Could you check a few things on this drawing? It's one solid part, dimensions in mm from its lowest x, y, z. A direction names the side the tool comes from. Give positions to 0.01 mm unless a question says otherwise; leave off trailing zeros. Loops run counter-clockwise (first coordinate to the right, second up) from the corner with the lowest first, then second, coordinate; pieces in that order, holes last. Notation, with made-up numbers: (16, -9) - (57, -9) arc R21 cw to (57, 28) - close; hole circle Ø5 at (11.5, 28). An arc over 180 degrees is marked (long way). Use CSV: the item, a comma, the result in double quotes.
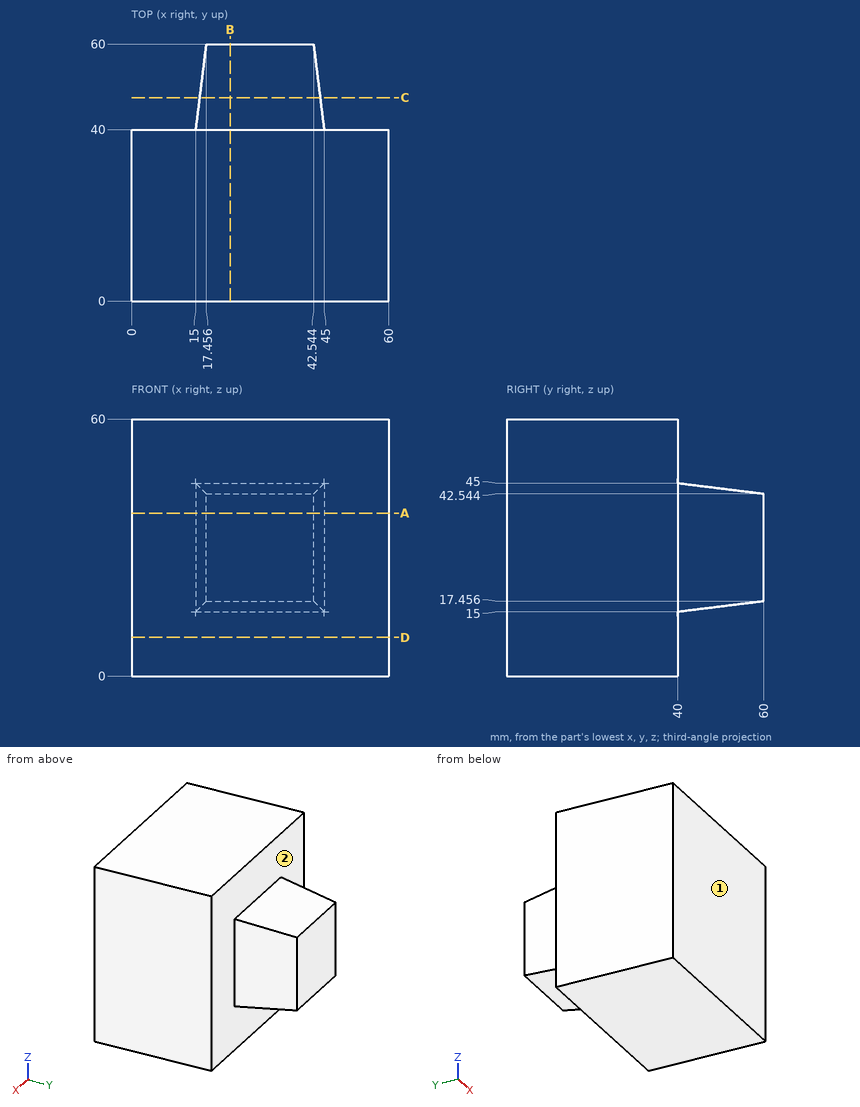
1) Which directions (+Z, -Z, +X, -X, +Y, -Y) give clear straight access to the entire face, cutting with the end or side of a thin tool? Please do the marked faces 1 and 2.
Answer below:
face 1,"+Z, -Z, +X, -X, -Y"
face 2,"+Y"
2) I need wall thicknesses on line 1 along Y through (x, z) = (39, 54.5); line 2 along X through (y, z) = (45, 21); line 3 along Z through (x, y) = (25.5, 51.5). Which ranges of each line are inside material? Lowest first, please.
Answer below:
line 1,"y = 0 to 40"
line 2,"x = 15.61 to 44.39"
line 3,"z = 16.41 to 43.59"
3) I'm going to push flat-ended pins straight in: P1, Ø2, axis at x = 38, y = 36.5, coming from the -Z side; P2, Ø8, axis at x = 27, y = 45.5, coming from the +Z side. Where does each tip first touch, or does it pass through?
Answer below:
P1,"stops at z = 0"
P2,"stops at z = 44.82"
4) Suppose I cut it at B-B (x = 23). Please give me the cut outline in (y, z), plus the area to 3 significant figures.
Answer below:
outline,"(0, 0) - (40, 0) - (40, 15) - (60, 17.46) - (60, 42.54) - (40, 45) - (40, 60) - (0, 60) - close"
area,"2,950 mm2"
5) Suppose I cut it at C-C (y = 47.5). Please give me the cut outline in (x, z).
Answer below:
outline,"(15.92, 15.92) - (44.08, 15.92) - (44.08, 44.08) - (15.92, 44.08) - close"
6) Suppose I cut it at A-A (z = 38). Please give me the cut outline in (x, y).
Answer below:
outline,"(0, 0) - (60, 0) - (60, 40) - (45, 40) - (42.54, 60) - (17.46, 60) - (15, 40) - (0, 40) - close"
7) Suppose I cut it at D-D (z = 9). Please give me the cut outline in (x, y), plus the area to 3 significant figures.
Answer below:
outline,"(0, 0) - (60, 0) - (60, 40) - (0, 40) - close"
area,"2,400 mm2"
